Geometry: final body of the model. Coordinates: model frame, mm. Face numbers are marked on the shaded views. A direction names the side the tool comes from. Give positions to 0.01 mm unless a question says otherwise; leave off trailing zeros. Order: outer loops, then holes, each group sorted by start corner. A loop starts at its lowest first (then second) coordinate and runs counter-clockwise, first axis right, second up. Notation, with made-up numbers: (-8, -34) - (46, -34) arc R20 ccw to (46, 4) - close; hole circle Ø7 at (77.25, 6.25). An arc over 180 degrees is marked (long way). Write item = value, one per line. Start each with the question number.
from build123d import *

# Parameters (mm, degrees)
ESBO_O1_R                = 3.5
ESBO_O1_R_2              = 2.5
RESSALTO_EXTRUS_O1_DEPTH = 6
RESSALTO_EXTRUS_O2_DEPTH = 6
PADR_OCIRCULAR1_COUNT    = 18


with BuildPart() as part:
    # Esboço1 → Ressalto-extrusão1 (new body)
    with BuildSketch(Plane.XY):
        Circle(ESBO_O1_R)
        Circle(ESBO_O1_R_2, mode=Mode.SUBTRACT)
    extrude(amount=RESSALTO_EXTRUS_O1_DEPTH)

    # Esboço1<3> → Ressalto-extrusão2 (add)
    with BuildSketch(Plane.XY):
        with BuildLine():
            ThreePointArc((0.3, 4.990991885), (0, 5), (-0.3, 4.990991885))
            Line((-0.3, 4.990991885), (-0.4, 3.47706773))
            ThreePointArc((-0.4, 3.47706773), (0, 3.5), (0.4, 3.47706773))
            Line((0.4, 3.47706773), (0.3, 4.990991885))
        make_face()
    ressalto_extrus_o2 = extrude(amount=RESSALTO_EXTRUS_O2_DEPTH)

    # PadrãoCircular1: Ressalto-extrusão2 ×18 about axis
    padr_ocircular1_axis = Axis((0, 0, 0), (0, 0, 1))
    for i in range(1, PADR_OCIRCULAR1_COUNT):
        add(ressalto_extrus_o2.rotate(padr_ocircular1_axis, i * 360 / PADR_OCIRCULAR1_COUNT))


solid = part.part
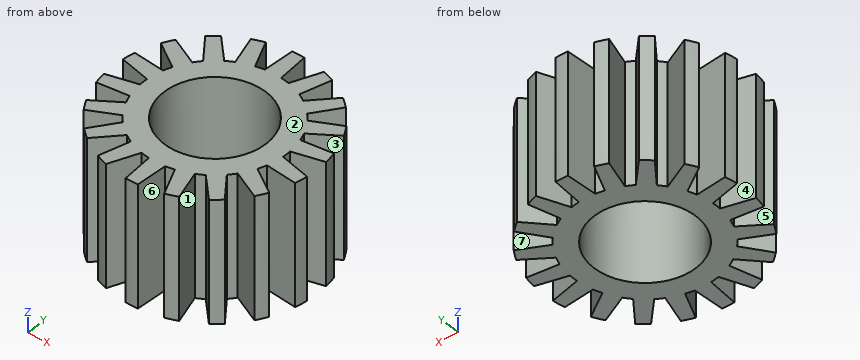
Q1. Section C-C, the plane x = 4. Return the cut outline in (y, z), then the cut area to 3 significant figures.
Q2. Set-up query: the marked faces 5, 6 and 7. Return all of +Z, -Z, +X, -X, +Y, -Y with unobstructed straight access to the full face (end or side cutting, diameter ignored); none if empty.
Q3. Material intervals for line 1 along Y through (x, z) = (-3, 5.3); line 2 along Y through (x, z) = (0, 4.2); line 3 along X through (y, z) = (1.5, 2.15), sorted ascending. Write a range as from..to.
Q4. Contact query for flat-ended pins moving along their axis: pin 1 (1.5 mm diameter, centred on y = 2, z = 1.5, fed in from +X); pin 2 (3 mm diameter, centred on y = 2, z = 4.5, fed in from -X). Output: stop coordinate, or through.
Q5. Section A-A, the plane y = 0. Return the cut outline in (x, z).
Q6. Pull-direction query (X, two-part tool) for the marked faces 1, 2, 3 and 4; classes: +X half, -X half, draft (parallel to the pull), parting line (faces both ways), or undercut.
Q7. Section B-B, the plane x = -1. Return the cut outline in (y, z).
The answers:
q1.outline = (-2.67, 0) - (-1.92, 0) - (-1.92, 6) - (-2.67, 6) - close; (-1.07, 0) - (-0.33, 0) - (-0.33, 6) - (-1.07, 6) - close; (0.33, 0) - (1.07, 0) - (1.07, 6) - (0.33, 6) - close; (1.92, 0) - (2.67, 0) - (2.67, 6) - (1.92, 6) - close
q1.area = 17.8 mm²
q2.face_5 = +Z, -Z, -X
q2.face_6 = +Z, -Z, -Y
q2.face_7 = +Z, -Z
q3.line_1 = -4..-3.03, -2.18..2.18, 3.03..4
q3.line_2 = -5..-2.5, 2.5..5
q3.line_3 = -3.37..-2, 2..3.37
q4.pin_1 = 4.47
q4.pin_2 = -4.97
q5.outline = (-3.5, 0) - (-2.5, 0) - (-2.5, 6) - (-3.5, 6) - close; (2.5, 0) - (3.5, 0) - (3.5, 6) - (2.5, 6) - close
q6.face_1 = undercut
q6.face_2 = draft
q6.face_3 = +X half
q6.face_4 = -X half
q7.outline = (-3.83, 0) - (-2.29, 0) - (-2.29, 6) - (-3.83, 6) - close; (2.29, 0) - (3.83, 0) - (3.83, 6) - (2.29, 6) - close
